from build123d import *

# Parameters (mm, degrees)
BOSS_EXTRUDE1_DEPTH = 5
SKETCH2_R           = 1.5
CUT_EXTRUDE1_DEPTH  = 5
SKETCH3_R           = 3
CUT_EXTRUDE2_DEPTH  = 5
SKETCH4_R           = 3
CUT_EXTRUDE3_DEPTH  = 10


with BuildPart() as part:
    # Sketch1 → Boss-Extrude1 (new body)
    with BuildSketch(Plane.XY):
        with BuildLine():
            Line((125, -20), (-125, -20))
            ThreePointArc((-125, -20), (-145, 0), (-125, 20))
            Line((-125, 20), (125, 20))
            ThreePointArc((125, 20), (145, 0), (125, -20))
        make_face()
    extrude(amount=BOSS_EXTRUDE1_DEPTH)

    # Sketch2 → Cut-Extrude1 (cut)
    with BuildSketch(Plane.XY.offset(5)):
        with Locations((-124.274977314, 13)):
            Circle(SKETCH2_R)
        with Locations((-111.274977314, 0)):
            Circle(SKETCH2_R)
        with Locations((-124.274977314, -13)):
            Circle(SKETCH2_R)
        with Locations((-137.274977314, 0)):
            Circle(SKETCH2_R)
        with Locations((125.216266839, 13)):
            Circle(SKETCH2_R)
        with Locations((138.216266839, 0)):
            Circle(SKETCH2_R)
        with Locations((125.216266839, -13)):
            Circle(SKETCH2_R)
        with Locations((112.216266839, 0)):
            Circle(SKETCH2_R)
    extrude(amount=-CUT_EXTRUDE1_DEPTH, mode=Mode.SUBTRACT)

    # Sketch3 → Cut-Extrude2 (cut)
    with BuildSketch(Plane(origin=(0, 0, 0), x_dir=(-1, 0, 0), z_dir=(0, 0, -1))):
        with Locations((-125.216266839, 0)):
            Circle(SKETCH3_R)
    extrude(amount=-CUT_EXTRUDE2_DEPTH, mode=Mode.SUBTRACT)

    # Sketch4 → Cut-Extrude3 (cut)
    with BuildSketch(Plane(origin=(0, 0, 0), x_dir=(-1, 0, 0), z_dir=(0, 0, -1))):
        with Locations((124.274977314, 0)):
            Circle(SKETCH4_R)
    extrude(amount=-CUT_EXTRUDE3_DEPTH, mode=Mode.SUBTRACT)


solid = part.part
CAD build for the part. Positions are in the model's coordinates, mm. Round coordinates to 2 decimals unless told otherwise and drop trailing zeros. Order: outer loops, then holes, each group sorted by start corner. A loop starts at its lowest first (then second) coordinate and runs counter-clockwise, first axis right, second up. Notation, with made-up numbers: (89, 61.25) - (145, 61.25) arc R7 cw to (145, 67.25) - close; hole circle Ø6 at (69.25, 66). An arc over 180 degrees is marked (long way). Return JSON: item names as keys, results as strings.
(1) Wall check: probe 1 along Y at (x, z) = (-124, 0.9); probe 2 along X at (y, z) = (6, 2.45); probe 3 along Y at (x, z) = (-126, 0.8). Give the ranges that are in metal, low to high. Write a range as from..to.
Answer key:
{"probe 1": "y = -20..-14.47, -11.53..-2.99, 2.99..11.53, 14.47..20", "probe 2": "x = -144.08..144.08", "probe 3": "y = -19.97..-2.45, 2.45..19.97"}
(2) Cut at A-A (z = 3.4). State how many separate pieces and enclosed holes the cut face has, then the cut area to 3 significant figures.
Answer key:
{"separate pieces": "1", "enclosed holes": "10", "area": "11,100 mm^2"}
(3) Pull direction X, two halves, no side cores. Call faces 1 (the face through (-121.894, -1.825, 2.465)), 2 (the face through (145, 0, 2)), 3 (the face through (2, 0, 0)): +X half, -X half, draft (parallel to the pull), parting line (faces both ways), or undercut.
Answer key:
{"face 1": "undercut", "face 2": "+X half", "face 3": "draft"}
(4) Cut at B-B (y = -17.5). Give the cut face in (x, z).
Answer key:
{"outline": "(-134.68, 0) - (134.68, 0) - (134.68, 5) - (-134.68, 5) - close"}
(5) Pin check, flat tip, straight feed: pin 1 Ø1.5 at (x, y) = (-110.5, 6) entering from -Z. Stop position of the tip, or through.
Answer key:
{"pin 1": "stops at z = 0"}
